Here's how the part is built. I have some questions about the finished solid (model axes, mm). A direction names the side the tool comes from. Round coordinates to 2 decimals unless told otherwise and drop trailing zeros. Write each loop counter-clockwise with the first axis right and the second up, starting at its lowest first coordinate (ties: lowest second). Pieces come first, ordered by that corner, then holes. Notation, with made-up numbers: (26, 12.25) -> (54, 12.25) arc R26 cw to (54, 36.25) -> close; hole circle Ø7 at (8, 70.25). An arc over 180 degrees is marked (long way). Answer in a Markdown table with one row per item.
from build123d import *

# Parameters (mm, degrees)
EXTRUDE_1_DEPTH     = 10
SKETCH_3_W          = 3
SKETCH_3_H          = 8
CUT_EXTRUDE_2_DEPTH = 10
EXTRUDE_2_DEPTH     = 2.5
CUT_EXTRUDE_3_DEPTH = 5
SKETCH_7_W          = 2
SKETCH_7_H          = 8.000466976
CUT_EXTRUDE_4_DEPTH = 2
SKETCH_8_W          = 2
SKETCH_8_H          = 8.002206322
CUT_EXTRUDE_5_DEPTH = 2


with BuildPart() as part:
    # 草圖1 → 填料-伸長1 (new body)
    with BuildSketch(Plane.XY):
        with BuildLine():
            Line((0, 0), (0, -27.033455112))
            ThreePointArc((0, -27.033455112), (3.346359716, -27.968396912), (6.692719433, -27.033455112))
            Line((6.692719433, -27.033455112), (6.692719433, 0))
            ThreePointArc((6.692719433, 0), (3.346359716, 0.689675236), (0, 0))
        make_face()
    extrude(amount=EXTRUDE_1_DEPTH)

    # 草圖3 → 除料-伸長2 (cut)
    with BuildSketch(Plane.XY.offset(10)):
        with Locations((3.5, -13.067229779)):
            Rectangle(SKETCH_3_W, SKETCH_3_H)
    extrude(amount=-CUT_EXTRUDE_2_DEPTH, mode=Mode.SUBTRACT)

    # 草圖4 → 填料-伸長2 (add, symmetric)
    with BuildSketch(Plane(origin=(0, -12.5, -0.092640319), x_dir=(1, 0, 0), z_dir=(0, 1, 0))):
        with BuildLine():
            Line((6.308695553, -9.676441633), (11.912423264, -9.676441633))
            ThreePointArc((11.912423264, -9.676441633), (13.672894686, -5.014177318), (11.912423264, -0.351913003))
            Line((11.912423264, -0.351913003), (6.308695553, -0.351913003))
            Line((6.308695553, -0.351913003), (6.308695553, -9.676441633))
        make_face()
    extrude(amount=EXTRUDE_2_DEPTH, both=True)

    # 草圖6 → 除料-伸長3 (cut)
    with BuildSketch(Plane(origin=(0, -10, 0), x_dir=(1, 0, 0), z_dir=(0, 1, 0))):
        with BuildLine():
            Line((6.692719433, -8.535251287), (11.039203193, -8.535251287))
            ThreePointArc((11.039203193, -8.535251287), (12.370150215, -4.897261986), (11.039203193, -1.259272684))
            Line((11.039203193, -1.259272684), (6.692719433, -1.259272684))
            Line((6.692719433, -1.259272684), (6.692719433, -8.535251287))
        make_face()
    extrude(amount=-CUT_EXTRUDE_3_DEPTH, mode=Mode.SUBTRACT)

    # 草圖7 → 除料-伸長4 (cut)
    with BuildSketch(Plane(origin=(0, 0, 0), x_dir=(-1, 0, 0), z_dir=(0, 0, -1))):
        with Locations((-1, -13.067463267)):
            Rectangle(SKETCH_7_W, SKETCH_7_H)
    extrude(amount=-CUT_EXTRUDE_4_DEPTH, mode=Mode.SUBTRACT)

    # 草圖8 → 除料-伸長5 (cut)
    with BuildSketch(Plane.XY.offset(10)):
        with Locations((1, -13.06833294)):
            Rectangle(SKETCH_8_W, SKETCH_8_H)
    extrude(amount=-CUT_EXTRUDE_5_DEPTH, mode=Mode.SUBTRACT)


solid = part.part
1) I want a section at D-D, the plane z = 7. List the corners of the cut face in (x, y) for me.
Response:
| item | result |
|---|---|
| outline | (0, -27.03) arc R6.46 ccw to (6.69, -27.03) -> (6.69, 0) arc R8.46 ccw to (0, 0) -> close; (11.96, -15) -> (13.36, -15) -> (13.36, -10) -> (11.96, -10) -> close; hole (2, -17.07) -> (5, -17.07) -> (5, -9.07) -> (2, -9.07) -> close |
2) I need wall thicknesses on line 1 (X direction, y = -14, z = 5); line 2 (Z direction, x = 9.25, y = -14.5); line 3 (X direction, y = -5.25, z = 1.5). Which ranges of each line are inside material? Lowest first, please. Write a range as [from, to].
Response:
| item | result |
|---|---|
| line 1 | x = [0, 2], [5, 6.69], [12.37, 13.67] |
| line 2 | z = [0.26, 1.26], [8.54, 9.58] |
| line 3 | x = [0, 6.69] |
3) I want a section at C-C, the plane x = 10. List the corners of the cut face in (y, z) for me, and give its area (3 significant figures).
Response:
| item | result |
|---|---|
| outline | (-15, 0.26) -> (-10, 0.26) -> (-10, 1.26) -> (-15, 1.26) -> close; (-15, 8.54) -> (-10, 8.54) -> (-10, 9.58) -> (-15, 9.58) -> close |
| area | 10.2 mm^2 |
4) I want a section at B-B, the plane z = 2.5. List the corners of the cut face in (x, y) for me, and give its area (3 significant figures).
Response:
| item | result |
|---|---|
| outline | (0, -27.03) arc R6.46 ccw to (6.69, -27.03) -> (6.69, 0) arc R8.46 ccw to (0, 0) -> close; (11.84, -15) -> (13.24, -15) -> (13.24, -10) -> (11.84, -10) -> close; hole (2, -17.07) -> (5, -17.07) -> (5, -9.07) -> (2, -9.07) -> close |
| area | 171 mm^2 |
5) Which directions (+Z, -Z, +X, -X, +Y, -Y) give clear straight access to the entire face, cutting with the end or side of a thin tool? Please do faces 5 (the face through (9, -12, 1.259)), 6 (the face through (9, -12, 9.584)), 7 (the face through (1, -17.069, 9)), 8 (the face through (12.5, -15, 5.6)).
Response:
| item | result |
|---|---|
| face 5 | +Y, -Y |
| face 6 | +Z, +X, +Y, -Y |
| face 7 | +Z, -X |
| face 8 | +Z, -Z, +X, -Y |
6) We'd pull the mould along X, two halves only. Please class faces 1 (the face through (3, -17.067, 5)), 2 (the face through (12.37, -12.46, 4.95)), 3 (the face through (0, -13, 5)), 4 (the face through (1, -17.068, 1)): +X half, -X half, draft (parallel to the pull), parting line (faces both ways), or undercut.
Response:
| item | result |
|---|---|
| face 1 | undercut |
| face 2 | undercut |
| face 3 | -X half |
| face 4 | draft |
7) I want a section at A-A, the plane y = -15.5. List the corners of the cut face in (x, z) for me, and give its area (3 significant figures).
Response:
| item | result |
|---|---|
| outline | (0, 2) -> (2, 2) -> (2, 8) -> (0, 8) -> close; (5, 0) -> (6.69, 0) -> (6.69, 10) -> (5, 10) -> close |
| area | 28.9 mm^2 |
8) For pin 1 (1.6 mm diameter, centred on x = 1.5, z = 9.5, fed in from +Y); pin 2 (3 mm diameter, centred on x = 9, z = 8.5, fed in from -Y); pin 3 (2 mm diameter, centred on x = 1.5, y = -11.5, fed in from -Z); pin 4 (2 mm diameter, centred on x = 10, z = 6.5, fed in from -Y), each with a flat end and sliding along its axis, tell me the tip position at first contact or that it passes through.
Response:
| item | result |
|---|---|
| pin 1 | stops at y = 0.62 |
| pin 2 | stops at y = -15 |
| pin 3 | stops at z = 2 |
| pin 4 | passes through |
